from build123d import *

# Parameters (mm, degrees)
BOSS_EXTRUDE1_DEPTH = 5
BOSS_EXTRUDE2_DEPTH = 20
CUT_EXTRUDE1_DEPTH  = 20
CUT_EXTRUDE2_DEPTH  = 20
CHAMFER1_SIZE       = 2


with BuildPart() as part:
    # Sketch1 → Boss-Extrude1 (new body)
    with BuildSketch(Plane(origin=(0, 0, 0), x_dir=(1, 0, 0), z_dir=(0, 1, 0))):
        Polygon((17.5, 12.5), (-12.5, -17.5), (-17.5, -17.5), (-17.5, 17.5), (17.5, 17.5), align=None)
    extrude(amount=BOSS_EXTRUDE1_DEPTH)

    # Sketch2 → Boss-Extrude2 (add)
    with BuildSketch(Plane(origin=(0, 5, 0), x_dir=(1, 0, 0), z_dir=(0, 1, 0))):
        Polygon((17.5, 17.5), (-17.5, 17.5), (-17.5, 12.5), (-17.5, -17.5), (-12.5, -17.5), (-8.5, -13.5), (-8.5, 6.5), (-12.5, 6.5), (-12.5, 12.5), (17.5, 12.5), align=None)
    extrude(amount=BOSS_EXTRUDE2_DEPTH)

    # Sketch3 → Cut-Extrude1 (cut)
    with BuildSketch(Plane(origin=(0, 0, -17.5), x_dir=(-1, 0, 0), z_dir=(0, 0, -1))):
        Polygon((-17.5, 5), (0, 25), (-17.5, 25), align=None)
    extrude(amount=-CUT_EXTRUDE1_DEPTH, mode=Mode.SUBTRACT)

    # Sketch4 → Cut-Extrude2 (cut)
    with BuildSketch(Plane.ZY.offset(17.5)):
        Polygon((17.5, 5), (0, 25), (17.5, 25), align=None)
    extrude(amount=-CUT_EXTRUDE2_DEPTH, mode=Mode.SUBTRACT)

    # Chamfer1
    chamfer1_edges = [part.edges().sort_by_distance(p)[0] for p in [
        (-17.5, 25, -8.75),
        (-8.75, 25, -17.5),
        (8.75, 15, -17.5),
        (-17.5, 15, 8.75),
    ]]
    chamfer(chamfer1_edges, length=CHAMFER1_SIZE)


solid = part.part
Can you work these out from the model? Positions are in its coordinate system, mm. A direction names the side the tool comes from. Coordinates: 2 decimals unless noted, no trailing zeros. Order: outer loops, then holes, each group sorted by start corner. A loop starts at its lowest first (then second) coordinate and runs counter-clockwise, first axis right, second up. Notation, with made-up numbers: (87.25, 11) -> (137.25, 11) arc R22 cw to (137.25, 39) -> close; hole circle Ø10 at (-19, -38). An arc over 180 degrees is marked (long way). Use one line per item in the form item = value.
Q1. We'd pull the mould along Z, two halves only. Please class faces 1 (the face through (-1, 13, -12.5)), 2 (the face through (8.89, 13.34, -16.49)), 3 (the face through (8.87, 14.86, -14.02)): released by +Z, released by -Z, zero draft, split by the parting line, or undercut.
From the geometry:
face_1 = undercut
face_2 = released by -Z
face_3 = zero draft
Q2. Will these pins go through, and if not, where does the flat tip stop? P1, Ø8, axis at y = 20, z = -7, coming from the +X side; P2, Ø12, axis at y = 10, z = -7.5, coming from the +X side; P3, Ø3, axis at y = 10, z = -10, coming from the +X side.
From the geometry:
P1 = -8.5
P2 = 16.03
P3 = -12.5
Q3. Which directions (+Z, -Z, +X, -X, +Y, -Y) give clear straight access to the entire face, cutting with the end or side of a thin tool? Please do faces 4 (the face through (-10, 15, -6.5)), 5 (the face through (-8.5, 13, 1)), 6 (the face through (2, 3, 3)).
From the geometry:
face_4 = +X, +Y
face_5 = +Z, +X, +Y
face_6 = +Z, +X, +Y, -Y
Q4. Imagine slicing it at A-A, the plane x = -7.5. List the corners of the cut face in (y, z) for me.
From the geometry:
outline = (0, -17.5) -> (23, -17.5) -> (25, -15.5) -> (25, -12.5) -> (5, -12.5) -> (5, 12.5) -> (0, 12.5) -> close
Q5. Imagine slicing it at C-C, the plane y = 6. List the corners of the cut face in (x, z) for me (3 decimals).
From the geometry:
outline = (-17.5, -17.5) -> (13.967, -17.5) -> (16.625, -15.5) -> (16.625, -12.5) -> (-12.5, -12.5) -> (-12.5, -6.5) -> (-8.5, -6.5) -> (-8.5, 13.5) -> (-11.625, 16.625) -> (-15.5, 16.625) -> (-17.5, 13.967) -> close
Q6. I need wall thicknesses on L1, parallel to X at y = 8, z = 12; L2, parallel to Z at x = 11, y = 8.75. Which ranges of each line are inside material? Lowest first, please.
From the geometry:
L1 = -17.5 to -8.5
L2 = -17.5 to -12.5
Q7. Imagine slicing it at D-D, the plane x = -13. List the corners of the cut face in (y, z) for me.
From the geometry:
outline = (0, -17.5) -> (23, -17.5) -> (25, -15.5) -> (25, 0) -> (5, 17.5) -> (0, 17.5) -> close
Q8. Imagine slicing it at B-B, the plane z = -11.5. List the corners of the cut face in (x, y) for me.
From the geometry:
outline = (-17.5, 0) -> (16.5, 0) -> (16.5, 5) -> (-12.5, 5) -> (-12.5, 25) -> (-15.5, 25) -> (-17.5, 23) -> close
